from build123d import *

# Parameters (mm, degrees)
SKETCH003_W = 87.46
SKETCH003_H = 76.45
SKETCH003_R = 31.7
PAD_DEPTH   = 38.21


with BuildPart() as female_shell:
    # Sketch003 → Pad (new body)
    with BuildSketch(Plane.XY):
        Rectangle(SKETCH003_W, SKETCH003_H)
        with Locations((0.217197, 0)):
            Circle(SKETCH003_R, mode=Mode.SUBTRACT)
    extrude(amount=PAD_DEPTH)


with BuildPart() as female_shell_1:
    # Body002 placement: moved
    add(female_shell.part.moved(Location((0, 0, 40))))


with BuildPart() as female_part:
    # Sketch002 → Revolution002 (revolve)
    with BuildSketch(Plane.XZ):
        with BuildLine():
            Line((0, 40), (31.7, 40))
            Line((31.7, 40), (31.7, 64.21))
            Line((28.525, 64.21), (31.7, 64.21))
            Line((28.525, 74.21), (28.525, 64.21))
            Line((28.525, 74.21), (25.35, 74.21))
            Line((25.35, 74.21), (25.35, 72.21))
            Line((25.35, 72.21), (22.175, 72.21))
            Line((22.175, 72.21), (22.175, 74.21))
            Line((22.175, 74.21), (19, 74.21))
            ThreePointArc((9, 74.21), (14, 69.21), (19, 74.21))
            Line((9, 74.21), (3.175, 74.21))
            Line((3.175, 72.21), (3.175, 74.21))
            Line((0, 72.21), (3.175, 72.21))
            Line((0, 72.21), (0, 40))
        make_face()
    revolve(axis=Axis((0, 0, 0), (0, 0, 1)))

    # Boolean: union female-shell
    add(female_shell_1.part)


solid = female_part.part
The listing builds one solid part. Answer for the finished solid, in the listing's coordinates (mm). A direction names the side the tool comes from. Round coordinates to 2 decimals unless told otherwise and drop trailing zeros. Write each loop counter-clockwise with the first axis right and the second up, starting at its lowest first coordinate (ties: lowest second). Pieces come first, ordered by that corner, then holes. Notation, with made-up numbers: M -20.75,53.25 L 2.25,53.25 A19 cw 2.25,57.25 Z; hole C 15.25,27.25 d11. An arc over 180 degrees is marked long. Write each question's results on one line, items separated by ' | '. Start each with the question number.
Item 1: A cutting plane is placed at C-C on y = -21. Write down the section's boundary in (x, z), and give its area (3 significant figures).
Item 2: A cutting plane is placed at D-D on x = -24. Write down the section's boundary in (y, z) (3 decimals).
Item 3: Straight lines are drawn through the part: L1, parallel to X at y = 0, z = 64; L2, parallel to X at y = 9, z = 70.5; L3, parallel to X at y = -25.5, z = 68.5. For each, find the intervals that lie inside material, in ascending order. Write a range as [from, to].
Item 4: For faces 1 (the face through (-20, 26, 78.21)), 2 (the face through (-6.184, -27.847, 69.14)), determine the directions among +Z, -Z, +X, -X, +Y, -Y from which every point of the face is accessible in a straight line to the end or side of a thin tool.
Item 5: A cutting plane is placed at B-B on x = 23.5. Write down the section's boundary in (y, z) (3 decimals), and give its area (3 significant figures).
Item 6: For a pull along X with two mould halves and no side action, classify faces 3 (the face through (-43.73, -1, 59)), 4 (the face through (-1, 1, 40)), 5 (the face through (0, 0, 72.21)), 6 (the face through (43.73, -1, 59)) as pulls with the +X half, pulls with the -X half, needs draft (parallel to the pull), parting line crosses it, or undercut.
Item 7: Flat-ended cylindrical pins translate along their axes: pin 1 Ø5.5 at (x, y) = (0, 0) entering from +Z; pin 2 Ø20 at (x, y) = (0.5, -3.5) entering from +Z. Find the tip coordinate at first contact, or state that the pin passes through.
Check sheet entries:
1) outline: M -43.73,40 L 23.75,40 L 23.75,64.21 L 19.3,64.21 L 19.3,74.21 L 14.2,74.21 L 14.2,72.21 L 7.12,72.21 L 7.12,74.21 L -7.12,74.21 L -7.12,72.21 L -14.2,72.21 L -14.2,74.21 L -19.3,74.21 L -19.3,64.21 L -23.53,64.21 L -23.53,78.21 L -43.73,78.21 Z; M 23.96,40 L 43.73,40 L 43.73,78.21 L 23.96,78.21 Z | area: 3,030 mm²
2) outline: M -38.225,40 L 38.225,40 L 38.225,78.21 L 20.455,78.21 L 20.455,64.21 L 15.417,64.21 L 15.417,74.21 L 8.162,74.21 L 8.162,72.21 L -8.162,72.21 L -8.162,74.21 L -15.417,74.21 L -15.417,64.21 L -20.455,64.21 L -20.455,78.21 L -38.225,78.21 Z
3) L1: [-43.73, 31.7], [31.92, 43.73] | L2: [-43.73, -30.18], [-27.07, -14.84], [-5.69, 5.69], [14.84, 27.07], [30.61, 43.73] | L3: [-43.73, -18.61], [-12.78, 12.78], [19.05, 43.73]
4) face 1: +Z, +X, -X, +Y, -Y | face 2: +Z
5) outline: M -38.225,40 L -21.513,40 L -21.513,78.21 L -38.225,78.21 Z; M -21.275,40 L 21.275,40 L 21.275,64.21 L 16.169,64.21 L 16.169,74.21 L 9.506,74.21 L 9.506,72.21 L -9.506,72.21 L -9.506,74.21 L -16.169,74.21 L -16.169,64.21 L -21.275,64.21 Z; M 21.513,40 L 38.225,40 L 38.225,78.21 L 21.513,78.21 Z | area: 2,590 mm²
6) face 3: pulls with the -X half | face 4: needs draft | face 5: undercut | face 6: pulls with the +X half
7) pin 1: z = 72.21 | pin 2: z = 74.21
